The model under review builds one solid part; all positions refer to its coordinate system, in mm. A direction names the side the tool comes from. Coordinates: 2 decimals unless noted, no trailing zeros. Write each loop counter-clockwise with the first axis right and the second up, starting at its lowest first coordinate (ties: lowest second). Pieces come first, ordered by that corner, then holes. Notation, with made-up numbers: (-40, 32) - (-3, 32) arc R21 ccw to (-3, 65) - close; hole circle Ø8 at (75, 24). An arc over 180 degrees is marked (long way). Put each result on its own line as item: value. Start each with the question number.
Item 1: For pin 1 (3 mm diameter, centred on x = 78, y = 5.5, fed in from +Z); pin 2 (6 mm diameter, centred on y = 13.5, z = 17, fed in from +X); pin 3 (6 mm diameter, centred on x = 72, z = 20, fed in from -Y); pin 4 (2 mm diameter, centred on y = 16, z = 5.5, fed in from +X), all flat-tipped, find the tip position at first contact; note any pin that passes through.
Item 2: Consider section B-B on x = 82. Give the boundary of the cut face in (y, z), then the cut area to 3 significant figures.
Item 3: Consider section C-C on z = 13.25. Give the boundary of the cut face in (x, y).
Item 4: Consider section D-D on x = 77.75. Give the boundary of the cut face in (y, z), then the cut area to 3 significant figures.
Item 5: To check wall thickness, follow L1, parallel to X at y = 3, z = 20; L2, parallel to Z at x = 76.25, y = 6.75; L3, parallel to Z at x = 73.25, y = 2.75. State the ranges of each line that lie inside material, in increasing order. Write a range as [from, to].
Item 6: Mouldability with a two-part tool opening along Y and no side actions: class faces 3 (the face through (67.999, 8, 11)), 4 (the face through (70.5, 18.485, 6.2)), 5 (the face through (81.619, 9.476, 1.268)), 6 (the face through (70.5, -1.515, 6.2)) as pulls with the +Y half, pulls with the -Y half, needs draft (parallel to the pull), parting line crosses it, or undercut.
Item 7: Consider section A-A on y = 10. Give the boundary of the cut face in (x, z).
Item 8: Machinability: for faces 1 (the face through (87.999, 8, 1)), 2 (the face through (70.499, 8, 15)), which of the approach directions +Z, -Z, +X, -X, +Y, -Y give a long, thin tool a straight path to every point of the face, cutting with its end or side? Answer none if there is none.
```python
from build123d import *

# Parameters (mm, degrees)
SKETCH2_W           = 20
SKETCH2_H           = 20
BOSS_EXTRUDE1_DEPTH = 2.5
SKETCH3_W           = 2.5
SKETCH3_H           = 20
BOSS_EXTRUDE2_DEPTH = 22.5
FILLET1_R           = 5
SKETCH4_R           = 1
CUT_EXTRUDE1_DEPTH  = 22.5


with BuildPart() as part:
    # Sketch2 → Boss-Extrude1 (new body)
    with BuildSketch(Plane.XY):
        with Locations((77.998956535, 8.484810347)):
            Rectangle(SKETCH2_W, SKETCH2_H)
    extrude(amount=BOSS_EXTRUDE1_DEPTH)

    # Sketch3 → Boss-Extrude2 (add)
    with BuildSketch(Plane.XY):
        with Locations((69.248956535, 8.484810347)):
            Rectangle(SKETCH3_W, SKETCH3_H)
    extrude(amount=BOSS_EXTRUDE2_DEPTH)

    # Fillet1
    fillet1_edges = [part.edges().sort_by_distance(p)[0] for p in [
        (70.498956535, 8.484810347, 2.5),
    ]]
    fillet(fillet1_edges, radius=FILLET1_R)

    # Sketch4 → Cut-Extrude1 (cut)
    with BuildSketch(Plane.XY.offset(2.5)):
        with Locations((81.748956535, 8.484810347)):
            Circle(SKETCH4_R)
    extrude(amount=-CUT_EXTRUDE1_DEPTH, mode=Mode.SUBTRACT)


solid = part.part
```
Report:
1. pin 1: z = 2.5
1. pin 2: x = 70.5
1. pin 3: y = -1.52
1. pin 4: x = 71.5
2. outline: (-1.52, 0) - (7.52, 0) - (7.52, 2.5) - (-1.52, 2.5) - close; (9.45, 0) - (18.48, 0) - (18.48, 2.5) - (9.45, 2.5) - close
2. area: 45.2 mm²
3. outline: (68, -1.52) - (70.5, -1.52) - (70.5, 18.48) - (68, 18.48) - close
4. outline: (-1.52, 0) - (18.48, 0) - (18.48, 2.5) - (-1.52, 2.5) - close
4. area: 50.0 mm²
5. L1: [68, 70.5]
5. L2: [0, 2.5]
5. L3: [0, 3.03]
6. face 3: needs draft
6. face 4: pulls with the +Y half
6. face 5: undercut
6. face 6: pulls with the -Y half
7. outline: (68, 0) - (88, 0) - (88, 2.5) - (75.5, 2.5) arc R5 cw to (70.5, 7.5) - (70.5, 22.5) - (68, 22.5) - close
8. face 1: +Z, -Z, +X, +Y, -Y
8. face 2: +Z, +X, +Y, -Y
